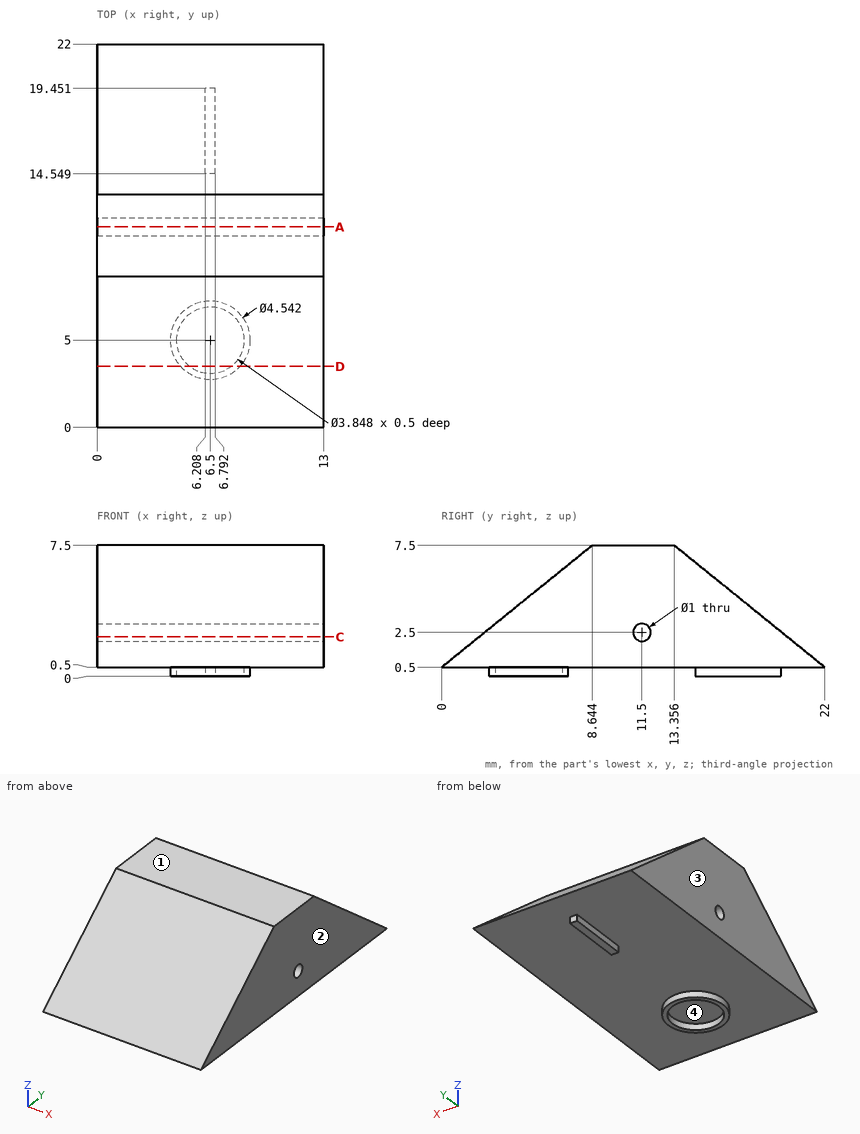
Part print with two shaded views. Sizes in mm from the minimum x, y, z corner. Round coordinates to 2 decimals unless told otherwise and drop trailing zeros. Write each loop counter-clockwise with the first axis right and the second up, starting at its lowest first coordinate (ties: lowest second). Pieces come first, ordered by that corner, then holes. Notation, with made-up numbers: M -3,38.25 L 53,38.25 A21 cw 53,74.25 Z; hole C 61,-23.5 d10. An arc over 180 degrees is marked long. Answer as CSV lines item,"result". Start each with the question number.
1) Drill centre lines: L1, parallel to Y at x = 6.5, z = 0.15; L2, parallel to Z at x = 12.75, y = 13.25; L3, parallel to Z at x = 10, y = 11.5. Where is each one in solid material? Low to high.
2) Band-saw the part on C-C (z = 2.25). List the corners of the cut face in (x, y).
3) Band-saw the part on A-A (y = 11.5). List the corners of the cut face in (x, z).
4) Drop flat-ended pins along their axis: pin 1 (3 mm diameter, centred on x = 4.5, z = 6.5, fed in from +Y); pin 2 (1.5 mm diameter, centred on x = 4.5, z = 2.5, fed in from +Y) (1 decimal); pin 3 (6 mm diameter, centred on x = 6.5, y = 5, fed in from +Z). Give the stop position or say it passes through.
5) Mould opens along X. For the marked faces 1, 2, 3 and 4 say: +X half, -X half, draft (parallel to the pull), parting line (faces both ways), or undercut.
6) Band-saw the part on D-D (y = 3.5). List the corners of the cut face in (x, z) (1 decimal).
Worked out:
1,L1,"2.73 to 3.08, 6.92 to 7.27, 14.55 to 19.45"
1,L2,"0.5 to 7.5"
1,L3,"0.5 to 2, 3 to 7.5"
2,outline,"M 0,2.16 L 13,2.16 L 13,11.07 L 0,11.07 Z; M 0,11.93 L 13,11.93 L 13,19.84 L 0,19.84 Z"
3,outline,"M 0,0.5 L 13,0.5 L 13,2 L 0,2 Z; M 0,3 L 13,3 L 13,7.5 L 0,7.5 Z"
4,pin 1,"y = 16.44"
4,pin 2,"y = 20.5"
4,pin 3,"z = 6.98"
5,face 1,"draft"
5,face 2,"+X half"
5,face 3,"-X half"
5,face 4,"undercut"
6,outline,"M 0,0.5 L 4.8,0.5 L 4.8,0 L 5.3,0 L 5.3,0.5 L 7.7,0.5 L 7.7,0 L 8.2,0 L 8.2,0.5 L 13,0.5 L 13,3.3 L 0,3.3 Z"
